```python
from build123d import *

# Parameters (mm, degrees)
BOSS_EXTRUDE1_DEPTH      = 50
BOSS_EXTRUDE1_DEPTH_BACK = 50
RIB1_REACH               = 222.474
SKETCH3_WALL_W           = 502.70716346
SKETCH3_WALL_H           = 10


with BuildPart() as part:
    # Sketch1 → Boss-Extrude1 (new, two sides: drawn at the far end of the back side and taken through both)
    with BuildSketch(Plane(origin=(0, 0, 0), x_dir=(0, 0, -1), z_dir=(1, 0, 0)).offset(-BOSS_EXTRUDE1_DEPTH_BACK)):
        Polygon((0, 0), (140, 0), (115.689255127, 137.873085422), (100.917138831, 135.268362757), (122.123696111, 15), (0, 15), align=None)
    extrude(amount=BOSS_EXTRUDE1_DEPTH + BOSS_EXTRUDE1_DEPTH_BACK)

    # Sketch3 wall → Rib1 (add, up to next)
    with BuildSketch(Plane(origin=(-50, 36.127729317, -93.545189355), x_dir=(0, -0.707106781187, 0.707106781187), z_dir=(0, 0.707106781187, 0.707106781187)), mode=Mode.PRIVATE) as rib1_sk1:
        with Locations((0, 5)):
            Rectangle(SKETCH3_WALL_W, SKETCH3_WALL_H)
    rib1_tool1 = extrude(rib1_sk1.sketch, amount=-RIB1_REACH, mode=Mode.PRIVATE) - part.part
    rib1 = rib1_tool1.solids().sort_by_distance((-50, 36.127729317, -93.545189355))[0]
    add(rib1)

    # Mirror1: Rib1 across plane
    add(rib1.mirror(Plane(origin=(0, 0, 0), x_dir=(0, 0, 1), z_dir=(1, 0, 0))))


solid = part.part
```
Geometry: final body of the model. Coordinates: model frame, mm. A direction names the side the tool comes from. Give positions to 0.01 mm unless a question says otherwise; leave off trailing zeros. Loops run counter-clockwise (first coordinate to the right, second up) from the corner with the lowest first, then second, coordinate; pieces in that order, holes last. Notation, with made-up numbers: (7.25, 36.25) -> (53.25, 36.25) arc R31 ccw to (53.25, 71.25) -> close; hole circle Ø5 at (7.25, 69). An arc over 180 degrees is marked (long way). Use one line per item in the form item = value.
Item 1: Section query C-C on y = 29.5. Output: boundary loops of the cut face in (x, z).
A:
outline = (-50, -134.8) -> (50, -134.8) -> (50, -86.92) -> (40, -86.92) -> (40, -119.57) -> (-40, -119.57) -> (-40, -86.92) -> (-50, -86.92) -> close
Item 2: Section query A-A on x = -42. Output: boundary loops of the cut face in (y, z).
A:
outline = (0, -140) -> (137.87, -115.69) -> (135.27, -100.92) -> (57.26, -114.67) -> (15, -72.42) -> (15, 0) -> (0, 0) -> close
Item 3: Section query B-B on z = -56. Output: boundary loops of the cut face in (x, y).
A:
outline = (-50, 0) -> (50, 0) -> (50, 15) -> (-50, 15) -> close
Item 4: Line query: probe 1 along Y at (x, z) = (-13, -55.5); probe 2 along Z at (x, y) = (27, 71.5); probe 3 along Z at (x, y) = (45, 123). Output: solid intervals per line, ascending.
A:
probe_1 = 0 to 15
probe_2 = -127.39 to -112.16
probe_3 = -118.31 to -103.08
Item 5: Section query D-D on x = -18. Output: boundary loops of the cut face in (y, z), and give its area (3 significant figures).
A:
outline = (0, -140) -> (137.87, -115.69) -> (135.27, -100.92) -> (15, -122.12) -> (15, 0) -> (0, 0) -> close
area = 3,930 mm^2
Item 6: Draft query along Y for faces 1 (the face through (-1, 0, -69)), 2 (the face through (40, 30, -101)), 3 (the face through (-0.7, 67.971, -128.015)), 4 (the face through (-1, 8, 0)). Return one class per face: pulls with the +Y half, pulls with the -Y half, needs draft (parallel to the pull), parting line crosses it, or undercut.
A:
face_1 = pulls with the -Y half
face_2 = undercut
face_3 = pulls with the +Y half
face_4 = needs draft
Item 7: Access query for faces 5 (the face through (-0.7, 75.98, -111.37)), 6 (the face through (-50, 36, -101)), 7 (the face through (-44.93, 36.42, -93.84)). Directions: +Z, -Z, +X, -X, +Y, -Y. A direction counts if a zero-diameter tool reaches every point of the face in a straight line with its end or side. Return the directions, or none.
A:
face_5 = +Z
face_6 = +Z, -Z, -X, +Y, -Y
face_7 = +Z, +X, -X
Item 8: Pin query (flat end, axial travel): P1, Ø12, axis at x = 23, y = 64, coming from the -Z side; P2, Ø8, axis at x = -28, z = -104, coming from the +Y side; P3, Ø2, axis at x = -15, y = 60, coming from the +Z side. Return the tip coordinate at first contact, or that it passes through.
A:
P1 = -129.77
P2 = 136.52
P3 = -114.01
